Work out the finished part from the listing and answer in its coordinate system (mm). Give positions to 0.01 mm unless a question says otherwise; leave off trailing zeros. Write each loop counter-clockwise with the first axis right and the second up, starting at its lowest first coordinate (ties: lowest second). Pieces come first, ordered by that corner, then holes. Notation, with made-up numbers: (33, 89) -> (82, 89) arc R25 ccw to (82, 104) -> close; hole circle Ø10 at (-35.5, 75). An arc over 180 degrees is marked (long way). Use a Markdown table: item, result. Add a question column.
Q1. Each of these flat-tipped pins is pushed along its axis until it touches: pin 1 Ø1 at (y, z) = (4, -26.5) entering from -X; pin 2 Ø5 at (x, z) = (45, -32.5) entering from -Y; pin 3 Ø3 at (x, y) = (43, 3) entering from -Z. Where does it stop, or does it pass through?
Q2. Section A-A, the plane z = -37.5 is taken. Give the vertices of the cut face in (x, y) (3 decimals).
Q3. Section B-B, the plane y = 1.7 is taken. Give the vertices of the cut face in (x, z) (3 decimals).
Q4. Section C-C, the plane x = 10 is taken. Give the vertices of the cut face in (y, z) (3 decimals).
Q5. Consider line 1 (Z direction, x = 40, y = 3.1) (3 decimals); line 2 (Z direction, x = 35, y = 3.75); line 3 (Z direction, x = 45, y = 4.05). Determine where each line is inside the solid, lowest interval first.
Q6. Section D-D, the plane z = -69 is taken. Give the vertices of the cut face in (x, y), plus the area to 3 significant figures.
from build123d import *

# Parameters (mm, degrees)
SKETCH1_W           = 50
SKETCH1_H           = 75
SKETCH1_R           = 1.875
SKETCH1_R_2         = 1.75
BOSS_EXTRUDE1_DEPTH = 5
SKETCH2_R           = 3
CUT_EXTRUDE1_DEPTH  = 2.5
FILLET1_R           = 30
FILLET2_R           = 10


with BuildPart() as part:
    # Sketch1 → Boss-Extrude1 (new body)
    with BuildSketch(Plane(origin=(0, 0, 0), x_dir=(1, 0, 0), z_dir=(0, 1, 0))):
        with Locations((25, 37.5)):
            Rectangle(SKETCH1_W, SKETCH1_H)
        with Locations((40, 65)):
            Circle(SKETCH1_R, mode=Mode.SUBTRACT)
        with Locations((40, 10)):
            Circle(SKETCH1_R, mode=Mode.SUBTRACT)
        with Locations((10, 37.5)):
            Circle(SKETCH1_R, mode=Mode.SUBTRACT)
        with Locations((45, 42.5)):
            Circle(SKETCH1_R_2, mode=Mode.SUBTRACT)
        with Locations((45, 32.5)):
            Circle(SKETCH1_R_2, mode=Mode.SUBTRACT)
        with Locations((35, 37.5)):
            Circle(SKETCH1_R_2, mode=Mode.SUBTRACT)
    extrude(amount=BOSS_EXTRUDE1_DEPTH)

    # Sketch2 → Cut-Extrude1 (cut)
    with BuildSketch(Plane.XZ):
        with Locations((45, -32.5)):
            Circle(SKETCH2_R)
        with Locations((45, -42.5)):
            Circle(SKETCH2_R)
        with Locations((35, -37.5)):
            Circle(SKETCH2_R)
    extrude(amount=-CUT_EXTRUDE1_DEPTH, mode=Mode.SUBTRACT)

    # Fillet1
    fillet1_edges = [part.edges().sort_by_distance(p)[0] for p in [
        (0, 2.5, -75),
        (0, 2.5, 0),
    ]]
    fillet(fillet1_edges, radius=FILLET1_R)

    # Fillet2
    fillet2_edges = [part.edges().sort_by_distance(p)[0] for p in [
        (50, 2.5, -75),
        (50, 2.5, 0),
    ]]
    fillet(fillet2_edges, radius=FILLET2_R)


solid = part.part
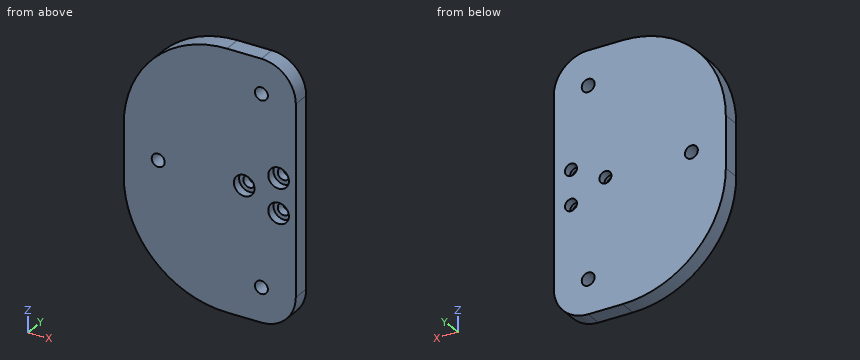
Result set:
| question | item | result |
|---|---|---|
| 1 | pin 1 | stops at x = 0.15 |
| 1 | pin 2 | stops at y = 2.5 |
| 1 | pin 3 | stops at z = -74.89 |
| 2 | outline | (0, 0) -> (8.125, 0) -> (8.125, 5) -> (0, 5) -> close; (11.875, 0) -> (32, 0) -> (32, 2.5) -> (33.25, 2.5) -> (33.25, 5) -> (11.875, 5) -> close; (36.75, 2.5) -> (38, 2.5) -> (38, 0) -> (50, 0) -> (50, 5) -> (36.75, 5) -> close |
| 3 | outline | (0, -45) arc R30 ccw to (30, -75) -> (40, -75) arc R10 ccw to (50, -65) -> (50, -10) arc R10 ccw to (40, 0) -> (30, 0) arc R30 ccw to (0, -30) -> close; hole circle Ø3.75 at (10, -37.5); hole circle Ø6 at (35, -37.5); hole circle Ø3.75 at (40, -65); hole circle Ø3.75 at (40, -10); hole circle Ø6 at (45, -42.5); hole circle Ø6 at (45, -32.5) |
| 4 | outline | (0, -67.361) -> (5, -67.361) -> (5, -39.375) -> (0, -39.375) -> close; (0, -35.625) -> (5, -35.625) -> (5, -7.639) -> (0, -7.639) -> close |
| 5 | line 1 | z = -75 to -66.875, -63.125 to -11.875, -8.125 to 0 |
| 5 | line 2 | z = -75 to -39.25, -35.75 to 0 |
| 5 | line 3 | z = -73.66 to -44.25, -40.75 to -34.25, -30.75 to -1.34 |
| 6 | outline | (12, 0) -> (49.17, 0) -> (49.17, 5) -> (12, 5) -> close |
| 6 | area | 186 mm2 |
